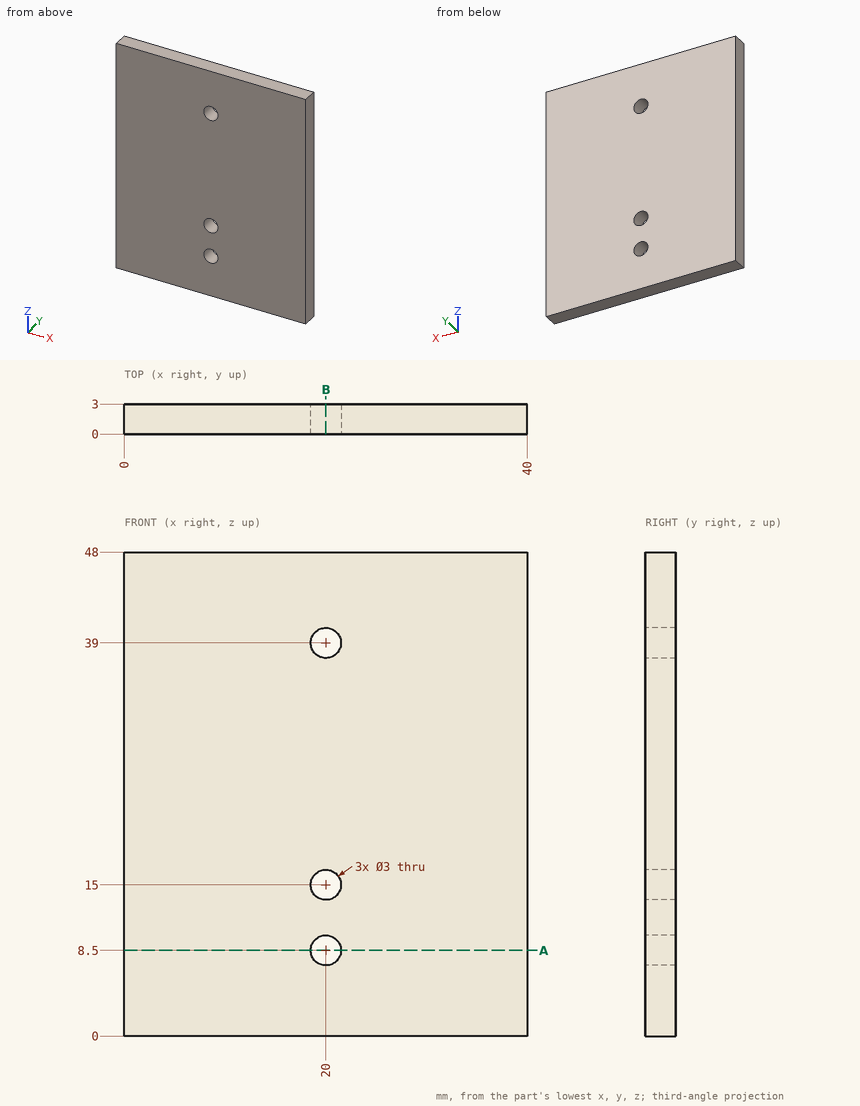
Answer from the drawing. Dimensions are ordinates in mm from the lowest x, y and z of the part. Give positions to 0.01 mm unless a question says otherwise; leave off trailing zeros. Loops run counter-clockwise (first coordinate to the right, second up) from the corner with the lowest first, then second, coordinate; pieces in that order, holes last.
Item 1: This flat-tipped pin is pushed along its axis until it touches: pin 1 Ø5 at (x, z) = (20, 39) entering from -Y. Where does it stop, or does it pass through?
Item 2: The part is cut by section B-B (x = 20). Write down the section's boundary in (y, z).
Item 3: The part is cut by section A-A (z = 8.5). Write down the section's boundary in (x, y), and give its area (3 significant figures).
Item 4: Find the intervals of material crossed by line 1 along Z through (x, y) = (20, 2.35); line 2 along Z through (x, y) = (19, 2.5); line 3 along X through (y, z) = (1.8, 9), in increasing order.
Taken from the geometry:
1. pin 1: stops at y = 0
2. outline: (0, 0) - (3, 0) - (3, 7) - (0, 7) - close; (0, 10) - (3, 10) - (3, 13.5) - (0, 13.5) - close; (0, 16.5) - (3, 16.5) - (3, 37.5) - (0, 37.5) - close; (0, 40.5) - (3, 40.5) - (3, 48) - (0, 48) - close
3. outline: (0, 0) - (18.5, 0) - (18.5, 3) - (0, 3) - close; (21.5, 0) - (40, 0) - (40, 3) - (21.5, 3) - close
3. area: 111 mm2
4. line 1: z = 0 to 7, 10 to 13.5, 16.5 to 37.5, 40.5 to 48
4. line 2: z = 0 to 7.38, 9.62 to 13.88, 16.12 to 37.88, 40.12 to 48
4. line 3: x = 0 to 18.59, 21.41 to 40
